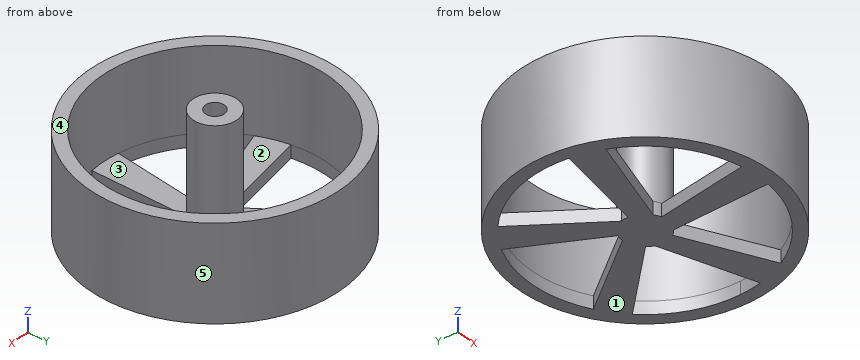
```python
from build123d import *

# Parameters (mm, degrees)
F0_R     = 20
F1_DEPTH = 15
F2_R     = 18
F3_DEPTH = 13
F4_R     = 3.5
F4_R_2   = 1.5
F5_DEPTH = 16
F7_DEPTH = 2


with BuildPart() as f1:
    # F0 (on Top) → F1 (new body)
    with BuildSketch(Plane.XY):
        Circle(F0_R)
    extrude(amount=F1_DEPTH)

    # F2 (on face) → F3 (cut)
    with BuildSketch(Plane.XY.offset(15)):
        Circle(F2_R)
    extrude(amount=-F3_DEPTH, mode=Mode.SUBTRACT)

    # F4 (on face) → F5 (join)
    with BuildSketch(Plane.XY.offset(2)):
        Circle(F4_R)
        Circle(F4_R_2, mode=Mode.SUBTRACT)
    extrude(amount=F5_DEPTH)

    # F6 (on face) → F7 (cut)
    with BuildSketch(Plane(origin=(0, 0, 0), x_dir=(1, 0, 0), z_dir=(0, 0, -1))):
        with BuildLine():
            ThreePointArc((-1.9313093683, 2.9189114622), (-1.42176068, 3.1982177175), (-0.8730234102, 3.3893701664))
            Line((-0.8730234102, 3.3893701664), (-2.7039568663, 17.7957471679))
            ThreePointArc((-2.7039568663, 17.7957471679), (-10.7932215062, 14.4050813784), (-16.3196684485, 7.5939727238))
            Line((-16.3196684485, 7.5939727238), (-1.9313093683, 2.9189114622))
        make_face()
        with BuildLine():
            ThreePointArc((-3.3728571828, -0.9347911128), (-3.4810340129, -0.3638711329), (-3.4932616532, 0.2170783785))
            Line((-3.4932616532, 0.2170783785), (-17.7603299302, 2.927572505))
            ThreePointArc((-17.7603299302, 2.927572505), (-17.0353353821, -5.813548694), (-12.2653521367, -13.1742603953))
            Line((-12.2653521367, -13.1742603953), (-3.3728571828, -0.9347911128))
        make_face()
        with BuildLine():
            ThreePointArc((-0.1532310099, -3.4966441423), (-0.7296366559, -3.4231024452), (-1.285931023, -3.2552083503))
            Line((-1.285931023, -3.2552083503), (-8.2725306819, -15.9864078553))
            ThreePointArc((-8.2725306819, -15.9864078553), (0.2648052303, -17.9980520665), (8.7392639441, -15.7361134247))
            Line((8.7392639441, -15.7361134247), (-0.1532310099, -3.4966441423))
        make_face()
        with BuildLine():
            ThreePointArc((18, 0), (17.9164345956, 1.7324466465), (17.6665142908, 3.448807448))
            Line((17.6665142908, 3.448807448), (3.2781552106, -1.2262538137))
            ThreePointArc((3.2781552106, -1.2262538137), (3.0300937601, -1.7517225252), (2.6985125738, -2.2289077794))
            Line((2.6985125738, -2.2289077794), (12.6476247957, -12.8077159176))
            ThreePointArc((12.6476247957, -12.8077159176), (16.6080890882, -6.9405602683), (18, 0))
        make_face()
        with BuildLine():
            Line((2.1792423504, 17.8675936482), (2.1792423504, 2.7387776066))
            ThreePointArc((2.1792423504, 2.7387776066), (2.6023375887, 2.3404783858), (2.9537035127, 1.8776675848))
            Line((2.9537035127, 1.8776675848), (16.0891926827, 8.0708041))
            ThreePointArc((16.0891926827, 8.0708041), (10.3647576432, 14.7163785966), (2.1792423504, 17.8675936482))
        make_face()
    extrude(amount=-F7_DEPTH, mode=Mode.SUBTRACT)


solid = f1.part
```
The listing builds one solid part. Answer for the finished solid, in the listing's coordinates (mm). Face numbers are marked on the shaded views. A direction names the side the tool comes from. Coordinates: 2 decimals unless noted, no trailing zeros. Write each loop counter-clockwise with the first axis right and the second up, starting at its lowest first coordinate (ties: lowest second). Pieces come first, ordered by that corner, then holes. Notation, with made-up numbers: (64.5, 56.25) -> (120.5, 56.25) arc R22 cw to (120.5, 93.25) -> close; hole circle Ø9 at (48, -20.5). An arc over 180 degrees is marked (long way). Write each question's results on one line, items separated by ' | '. Start each with the question number.
1) For a pull along X with two mould halves and no side action, classify the marked faces 3, 4 and 5 as +X half, -X half, draft (parallel to the pull), parting line (faces both ways), or undercut.
2) Flat-ended cylindrical pins translate along their axes: pin 1 Ø7.5 at (x, y) = (13.5, -5) entering from +Z; pin 2 Ø1 at (y, z) = (-7.5, 1) entering from +X (3 decimals); pin 3 Ø6 at (y, z) = (-14, 9) entering from -X. Find the tip coordinate at first contact, or state that the pin passes through.
3) A cutting plane is placed at A-A (z = 1.5). Determine the outline of the cut face in (x, y).
4) A cutting plane is placed at C-C (x = 8). Determine the outline of the cut face in (y, z).
5) A cutting plane is placed at D-D (z = 8.5). Determine the outline of the cut face in (x, y), then the cut area to 3 significant figures.
6) A tool of negligible diameter and unlimited length cuts with its end or side. For the marked faces 1 and 2, from which of +Z, -Z, +X, -X, +Y, -Y can it reach the whole face along a straight path? Write none if from no direction.
7) Straight lines are drawn through the part: probe 1 along Y at (x, z) = (0, 9); probe 2 along X at (y, z) = (-3, 8); probe 3 along Y at (x, z) = (-15, 8.25). For each, find the intervals that lie inside material, in ascending order.
8) A cutting plane is placed at B-B (y = 17). Determine the outline of the cut face in (x, z).
Values follow:
1) face 3: undercut | face 4: draft | face 5: parting line
2) pin 1: z = 15 | pin 2: x = 18.735 | pin 3: x = -16.7
3) outline: circle Ø40 at (0, 0); hole (-17.76, -2.93) -> (-3.49, -0.22) arc R3.5 cw to (-3.37, 0.93) -> (-12.27, 13.17) arc R18 ccw to start; hole (-16.32, -7.59) arc R18 ccw to (-2.7, -17.8) -> (-0.87, -3.39) arc R3.5 cw to (-1.93, -2.92) -> close; hole (-8.27, 15.99) -> (-1.29, 3.26) arc R3.5 cw to (-0.15, 3.5) -> (8.74, 15.74) arc R18 ccw to start; hole (2.18, -17.87) arc R18 ccw to (16.09, -8.07) -> (2.95, -1.88) arc R3.5 cw to (2.18, -2.74) -> close; hole (2.7, 2.23) arc R3.5 cw to (3.28, 1.23) -> (17.67, -3.45) arc R18 ccw to (12.65, 12.81) -> close
4) outline: (-18.33, 0) -> (-16.12, 0) -> (-16.12, 15) -> (-18.33, 15) -> close; (-4.26, 0) -> (-0.31, 0) -> (-0.31, 2) -> (-4.26, 2) -> close; (7.87, 0) -> (14.72, 0) -> (14.72, 2) -> (7.87, 2) -> close; (16.12, 0) -> (18.33, 0) -> (18.33, 15) -> (16.12, 15) -> close
5) outline: circle Ø40 at (0, 0); circle Ø7 at (0, 0); hole circle Ø36 at (0, 0); hole circle Ø3 at (0, 0) | area: 270 mm²
6) face 1: -Z, +X, -X, +Y, -Y | face 2: +Z
7) probe 1: -20 to -18, -3.5 to -1.5, 1.5 to 3.5, 18 to 20 | probe 2: -19.77 to -17.75, -1.8 to 1.8, 17.75 to 19.77 | probe 3: -13.23 to -9.95, 9.95 to 13.23
8) outline: (-10.54, 0) -> (-5.92, 0) -> (-5.92, 15) -> (-10.54, 15) -> close; (5.92, 0) -> (10.54, 0) -> (10.54, 15) -> (5.92, 15) -> close
